Study the drawing (mm; zero at the part's minimum x, y, z) and answer. Round coordinates to 2 decimals unless told otherwise and drop trailing zeros. Write each loop counter-clockwise with the first axis right and the second up, starting at its lowest first coordinate (ties: lowest second). Pieces come first, ordered by that corner, then holes. Notation, with made-up numbers: (1, 68) -> (15, 68) arc R21 ccw to (15, 74) -> close; hole circle Ø3 at (-23, -34.75). An arc over 180 degrees is marked (long way). Write each question's results on one line, items separated by ' | '. Start each with the question number.
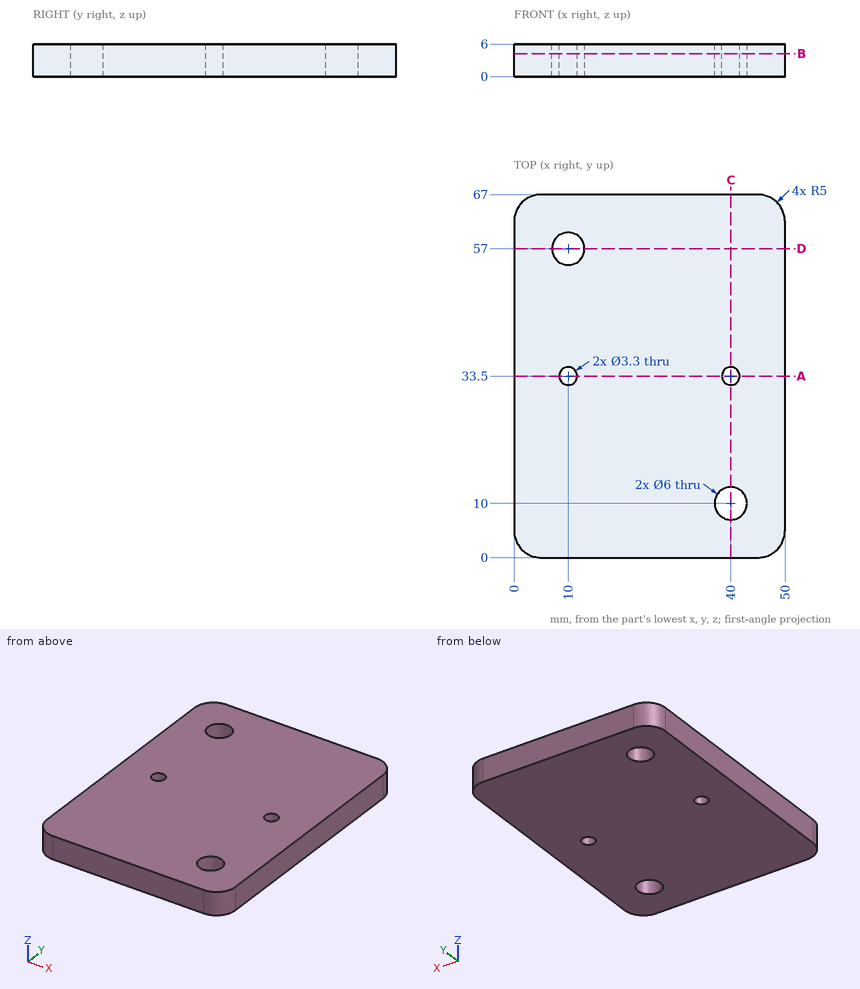
Q1. The part is cut by section A-A, the plane y = 33.5. Write down the section's boundary in (x, z).
Q2. The part is cut by section D-D, the plane y = 57. Write down the section's boundary in (x, z).
Q3. The part is cut by section C-C, the plane x = 40. Write down the section's boundary in (y, z), then the cut area to 3 significant figures.
Q4. Each of these flat-tipped pins is pushed along its axis until it touches: pin 1 (2 mm diameter, centred on x = 27, z = 3.5, fed in from -Y); pin 2 (3.5 mm diameter, centred on x = 10, y = 57, fed in from -Z). Where does it stop, or does it pass through?
Q5. The part is cut by section B-B, the plane z = 4.2. Write down the section's boundary in (x, y), then the cut area to 3 significant figures.
Q6. Find the intervals of material crossed by line 1 (Y direction, x = 40, z = 2.55); line 2 (Y direction, x = 10, z = 3.1); line 3 (X direction, y = 33.5, z = 4.15), in increasing order.
Answers follow:
1) outline: (0, 0) -> (8.35, 0) -> (8.35, 6) -> (0, 6) -> close; (11.65, 0) -> (38.35, 0) -> (38.35, 6) -> (11.65, 6) -> close; (41.65, 0) -> (50, 0) -> (50, 6) -> (41.65, 6) -> close
2) outline: (0, 0) -> (7, 0) -> (7, 6) -> (0, 6) -> close; (13, 0) -> (50, 0) -> (50, 6) -> (13, 6) -> close
3) outline: (0, 0) -> (7, 0) -> (7, 6) -> (0, 6) -> close; (13, 0) -> (31.85, 0) -> (31.85, 6) -> (13, 6) -> close; (35.15, 0) -> (67, 0) -> (67, 6) -> (35.15, 6) -> close | area: 346 mm^2
4) pin 1: y = 0 | pin 2: through
5) outline: (0, 5) arc R5 ccw to (5, 0) -> (45, 0) arc R5 ccw to (50, 5) -> (50, 62) arc R5 ccw to (45, 67) -> (5, 67) arc R5 ccw to (0, 62) -> close; hole circle Ø6 at (10, 57); hole circle Ø3.3 at (10, 33.5); hole circle Ø6 at (40, 10); hole circle Ø3.3 at (40, 33.5) | area: 3,250 mm^2
6) line 1: 0 to 7, 13 to 31.85, 35.15 to 67 | line 2: 0 to 31.85, 35.15 to 54, 60 to 67 | line 3: 0 to 8.35, 11.65 to 38.35, 41.65 to 50
